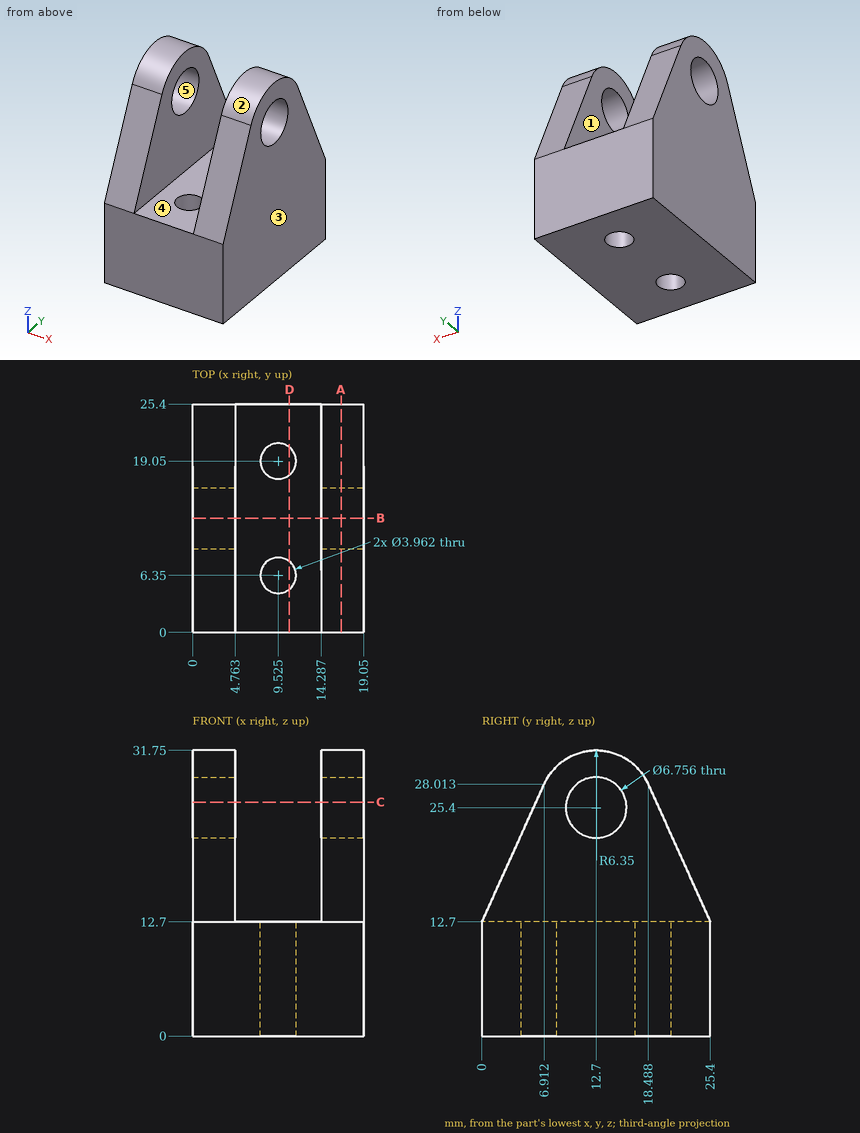
Could you check a few things on this drawing? It's one solid part, dimensions in mm from its lowest x, y, z. A direction names the side the tool comes from. Give positions to 0.01 mm unless a question says otherwise; leave off trailing zeros. Order: outer loops, then holes, each group sorted by start corner. A loop starts at its lowest first (then second) coordinate and runs counter-clockwise, first axis right, second up. Notation, with made-up numbers: (25, 42) - (37, 42) arc R20 ccw to (37, 75) - close; hole circle Ø9 at (30, -4). An arc over 180 degrees is marked (long way). One line per item, written item: value. Start each with the question number.
1. Imagine slicing it at B-B on y = 12.7. List the corners of the cut face in (x, z) for me.
2. For P1, Ø3, axis at x = 9.525, y = 6.35, coming from the -Z side; P2, Ø1, axis at x = 5.5, y = 11, coming from the +Z side; P3, Ø5, axis at x = 7, z = 19.5, coming from the +Y side (1 decimal), each with a flat end and sliding along its axis, tell me the tip position at first contact or that it passes through.
3. Thinking about a two-plate mould opening in X: for the marked faces 3, 4 and 5, which applies, +X half, -X half, draft (parallel to the pull), parting line (faces both ways), or undercut?
4. Imagine slicing it at D-D on x = 10.75. List the corners of the cut face in (y, z) for me.
5. Imagine slicing it at A-A on x = 16.5. List the corners of the cut face in (y, z) for me.
6. For the marked faces 1 and 2, which set-ups out of +Z, -Z, +X, -X, +Y, -Y let a thin tool reach every point of the face, with its end or its side?
7. If I drill on probe 1 along X at (y, z) = (19.05, 6.25); probe 2 along X at (y, z) = (19, 21); probe 3 along Z at (x, y) = (1, 12.5), over which ranges is the centre line in solid material (lowest first)?
8. Imagine slicing it at C-C on z = 26. Give the number of separate pieces and of enclosed holes in the cut face.
Values:
1. outline: (0, 0) - (19.05, 0) - (19.05, 22.02) - (14.29, 22.02) - (14.29, 12.7) - (4.76, 12.7) - (4.76, 22.02) - (0, 22.02) - close; (0, 28.78) - (4.76, 28.78) - (4.76, 31.75) - (0, 31.75) - close; (14.29, 28.78) - (19.05, 28.78) - (19.05, 31.75) - (14.29, 31.75) - close
2. P1: through
2. P2: z = 12.7
2. P3: y = 22.8
3. face 3: +X half
3. face 4: undercut
3. face 5: draft
4. outline: (0, 0) - (4.79, 0) - (4.79, 12.7) - (0, 12.7) - close; (7.91, 0) - (17.49, 0) - (17.49, 12.7) - (7.91, 12.7) - close; (20.61, 0) - (25.4, 0) - (25.4, 12.7) - (20.61, 12.7) - close
5. outline: (0, 0) - (25.4, 0) - (25.4, 12.7) - (18.49, 28.01) arc R6.35 ccw to (6.91, 28.01) - (0, 12.7) - close; hole circle Ø6.76 at (12.7, 25.4)
6. face 1: +Z, +Y, -Y
6. face 2: +Z, +X, -X
7. probe 1: 0 to 7.54, 11.51 to 19.05
7. probe 2: 0 to 4.76, 14.29 to 19.05
7. probe 3: 0 to 22.03, 28.77 to 31.75
8. separate pieces: 4
8. enclosed holes: 0
